Could you check a few things on this drawing? It's one solid part, dimensions in mm from its lowest x, y, z. Coordinates: 2 decimals unless noted, no trailing zeros. Write each loop counter-clockwise with the first axis right and the second up, starting at its lowest first coordinate (ties: lowest second). Pieces come first, ordered by that corner, then holes. Notation, with made-up numbers: (64.25, 48) - (119.25, 48) arc R24 cw to (119.25, 78) - close; hole circle Ø9 at (-23.75, 26.5). An arc over 180 degrees is marked (long way). Use one line per item in the form item = value. Start each with the question number.
(1) If we section it at B-B on y = 69: Please give me the cut outline in (x, z).
(2) For pin 1 Ø6 at (y, z) = (27.5, 4) entering from +X; pin 2 Ø6 at (y, z) = (12.5, 1.5) entering from -X; pin 3 Ø2 at (y, z) = (52.5, 13.5) entering from +X (1 decimal), each with a flat end and sliding along its axis, tell me the tip position at first contact or that it passes through.
(3) If we section it at C-C on z = 12.5: Please give me the cut outline in (x, y) (1 decimal), then the cut area to 3 significant figures.
(4) If we section it at A-A on x = 203.5: Please give me the cut outline in (y, z), then the cut area to 3 significant figures.
(5) If I drill on probe 1 along X at (y, z) = (97.5, 1.25) (1 decimal); probe 2 along X at (y, z) = (17.5, 7) (1 decimal); probe 3 along Y at (x, z) = (162, 8.5), over which ranges is the centre line in solid material (lowest first)? Write a range as from..to.
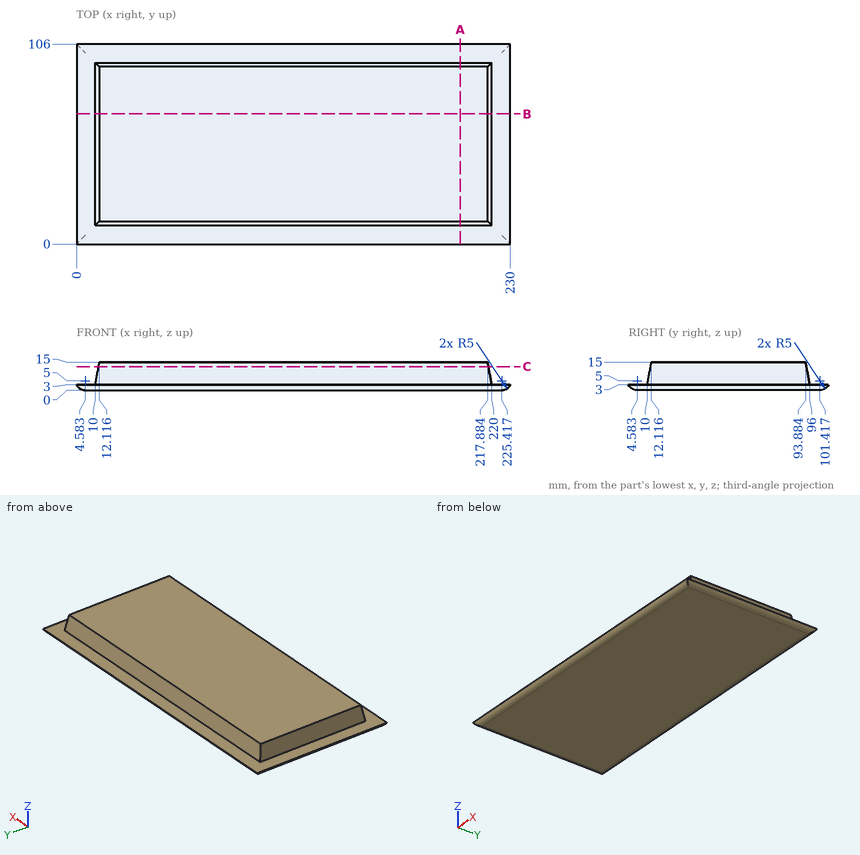
Reported:
q1.outline = (0, 3) arc R5 ccw to (4.58, 0) - (225.42, 0) arc R5 ccw to (230, 3) - (220, 3) - (217.88, 15) - (12.12, 15) - (10, 3) - close
q2.pin_1 = 230
q2.pin_2 = 0
q2.pin_3 = 218.3
q3.outline = (11.7, 11.7) - (218.3, 11.7) - (218.3, 94.3) - (11.7, 94.3) - close
q3.area = 17,100 mm2
q4.outline = (0, 3) arc R5 ccw to (4.58, 0) - (101.42, 0) arc R5 ccw to (106, 3) - (96, 3) - (93.88, 15) - (12.12, 15) - (10, 3) - close
q4.area = 1,320 mm2
q5.probe_1 = 1.3..228.7
q5.probe_2 = 10.7..219.3
q5.probe_3 = 10.97..95.03
